```python
from build123d import *

# Parameters (mm, degrees)
SKETCH1_W           = 14.6
SKETCH1_H           = 90
BOSS_EXTRUDE1_DEPTH = 5
FILLET1_R           = 5
SKETCH6_W           = 4
SKETCH6_H           = 25
CUT_EXTRUDE1_DEPTH  = 52.510096098
SKETCH7_W           = 2.5
SKETCH7_H           = 25
CUT_EXTRUDE2_DEPTH  = 52.355233424
FILLET4_R           = 2
SKETCH8_W           = 8
SKETCH8_H           = 20
CUT_EXTRUDE3_DEPTH  = 52.510096098


with BuildPart() as part:
    # Sketch1 → Boss-Extrude1 (new, symmetric)
    with BuildSketch(Plane.XY):
        with Locations((0, 5)):
            Rectangle(SKETCH1_W, SKETCH1_H)
    extrude(amount=BOSS_EXTRUDE1_DEPTH, both=True)

    # Fillet1
    fillet1_edges = [part.edges().sort_by_distance(p)[0] for p in [
        (7.3, -40, 0),
        (-7.3, -40, 0),
    ]]
    fillet(fillet1_edges, radius=FILLET1_R)

    # Sketch4 → Cut-Revolve2 (revolve, cut)
    with BuildSketch(Plane.XY):
        with BuildLine():
            Line((-7.3, -32), (-5.3, -32))
            ThreePointArc((-5.3, -32), (-5.885786438, -30.585786438), (-7.3, -30))
            Line((-7.3, -30), (-7.3, -32))
        make_face()
        with BuildLine():
            Line((7.3, -32), (5.3, -32))
            ThreePointArc((5.3, -32), (5.885786438, -30.585786438), (7.3, -30))
            Line((7.3, -30), (7.3, -32))
        make_face()
    revolve(axis=Axis((-17.666251228, -32, 0), (1, 0, 0)), mode=Mode.SUBTRACT)

    # Sketch6 → Cut-Extrude1 (cut, through all)
    with BuildSketch(Plane.XY.offset(5)):
        with Locations((-5.3, 37.5)):
            Rectangle(SKETCH6_W, SKETCH6_H)
        with Locations((5.3, 37.5)):
            Rectangle(SKETCH6_W, SKETCH6_H)
    extrude(amount=-CUT_EXTRUDE1_DEPTH, mode=Mode.SUBTRACT)

    # Sketch7 → Cut-Extrude2 (cut, through all)
    with BuildSketch(Plane(origin=(3.3, 0, 0), x_dir=(0, 0, -1), z_dir=(1, 0, 0))):
        with Locations((-3.75, 37.5)):
            Rectangle(SKETCH7_W, SKETCH7_H)
        with Locations((3.75, 37.5)):
            Rectangle(SKETCH7_W, SKETCH7_H)
    extrude(amount=-CUT_EXTRUDE2_DEPTH, mode=Mode.SUBTRACT)

    # Fillet4
    fillet4_edges = [part.edges().sort_by_distance(p)[0] for p in [
        (0, 50, 2.5),
        (0, 50, -2.5),
    ]]
    fillet(fillet4_edges, radius=FILLET4_R)

    # Sketch8 → Cut-Extrude3 (cut, through all)
    with BuildSketch(Plane(origin=(0, 0, -5), x_dir=(-1, 0, 0), z_dir=(0, 0, -1))):
        with Locations((0, -30)):
            Rectangle(SKETCH8_W, SKETCH8_H)
    extrude(amount=-CUT_EXTRUDE3_DEPTH, mode=Mode.SUBTRACT)


solid = part.part
```
Model file for the job. Use its own axes, mm. A direction names the side the tool comes from. Give positions to 0.01 mm unless a question says otherwise; leave off trailing zeros. Loops run counter-clockwise (first coordinate to the right, second up) from the corner with the lowest first, then second, coordinate; pieces in that order, holes last. Notation, with made-up numbers: (75.5, 44) -> (133.5, 44) arc R18 cw to (133.5, 66) -> close; hole circle Ø2 at (-9, 51.25). An arc over 180 degrees is marked (long way). Write each question's results on one line, items separated by ' | '.
(1) Pull direction X, two halves, no side cores. Call faces 1 (the flat face through (0, 36, -2.5)), 2 (the flat face through (4, -30, 0)), 3 (the flat face through (-3.3, 37, 0)): released by +X, released by -X, zero draft, split by the parting line, or undercut.
Geometry results:
face 1: zero draft | face 2: undercut | face 3: released by -X
(2) Tool access for faces 4 (the flat face through (0, -20, 0)), 5 (the flat face through (3.3, 37, 0)), 6 (the flat face through (0, 36, 2.5)), 7 (the flat face through (-7.3, -5, 0)): list every direction of +Z, -Z, +X, -X, +Y, -Y with a clear straight run to the whole face (end or side of a thin tool).
Geometry results:
face 4: +Z, -Z, -Y | face 5: +Z, -Z, +X, +Y | face 6: +Z, +X, -X, +Y | face 7: +Z, -Z, -X, +Y, -Y
(3) Cut at B-B on z = 3.5. List the corners of the cut face in (x, y), and give its area (3 significant figures).
Geometry results:
outline: (-7.3, -35) arc R5 ccw to (-4, -39.7) -> (-4, -20) -> (4, -20) -> (4, -39.7) arc R5 ccw to (7.3, -35) -> (7.3, 25) -> (-7.3, 25) -> close | area: 779 mm²
(4) Cut at D-D on x = -6.25. List the corners of the cut face in (y, z).
Geometry results:
outline: (-38.07, -5) -> (25, -5) -> (25, 5) -> (-38.07, 5) -> close; hole circle Ø3.4 at (-32, 0)
(5) Cut at A-A on y = -21. List the corners of the cut face in (x, z), and give its area (3 significant figures).
Geometry results:
outline: (-7.3, -5) -> (-4, -5) -> (-4, 5) -> (-7.3, 5) -> close; (4, -5) -> (7.3, -5) -> (7.3, 5) -> (4, 5) -> close | area: 66.0 mm²
(6) Cut at C-C on x = -1.5. List the corners of the cut face in (y, z), and give its area (3 significant figures).
Geometry results:
outline: (-20, -5) -> (25, -5) -> (25, -2.5) -> (48, -2.5) arc R2 ccw to (50, -0.5) -> (50, 0.5) arc R2 ccw to (48, 2.5) -> (25, 2.5) -> (25, 5) -> (-20, 5) -> close | area: 573 mm²
(7) Flat gauge pins, fed straight in: pin 1 Ø2.5 at (y, z) = (37, 0.5) entering from +X; pin 2 Ø5.5 at (x, y) = (-1, 41.5) entering from -Z; pin 3 Ø2 at (x, z) = (1.5, -2.5) entering from -Y. Where does each tip first touch, or does it go through?
Geometry results:
pin 1: stops at x = 3.3 | pin 2: stops at z = -2.5 | pin 3: stops at y = -20
(8) Probe line 1 along X through (y, z) = (-27, -3.75); line 2 along Y through (x, z) = (1.25, -0.5); line 3 along X through (y, z) = (33, 0.25). List the from-to ranges inside material, lowest first.
Geometry results:
line 1: x = -7.3 to -4, 4 to 7.3 | line 2: y = -20 to 50 | line 3: x = -3.3 to 3.3
